from build123d import *

# Parameters (mm, degrees)
BOSS_EXTRU_1_DEPTH = 50
CONG_1_R           = 0.75
CONG_2_R           = 0.25
CONG_3_R           = 0.25


with BuildPart() as part:
    # Esquisse1 → Boss.-Extru.1 (new body)
    with BuildSketch(Plane.XY):
        Polygon((3.2, 0), (0, 0), (0, 8), (-2, 8), (-2, 0), (-2, -2), (5.2, -2), (5.2, 0), (5.2, 8), (3.2, 8), align=None)
    extrude(amount=BOSS_EXTRU_1_DEPTH)

    # Congé1
    cong_1_edges = [part.edges().sort_by_distance(p)[0] for p in [
        (5.2, 8, 25),
        (-2, 8, 25),
    ]]
    fillet(cong_1_edges, radius=CONG_1_R)

    # Congé2
    cong_2_edges = [part.edges().sort_by_distance(p)[0] for p in [
        (3.2, 8, 25),
        (0, 8, 25),
    ]]
    fillet(cong_2_edges, radius=CONG_2_R)

    # Congé3
    cong_3_edges = [part.edges().sort_by_distance(p)[0] for p in [
        (1.6, 0, 0),
        (5.2, 2.625, 0),
        (0, 3.875, 0),
        (5.2, 2.625, 50),
        (-2, 2.625, 0),
        (-2, 2.625, 50),
        (3.95, 8, 0),
        (4.980330086, 7.780330086, 0),
        (-1.780330086, 7.780330086, 0),
        (3.95, 8, 50),
        (4.980330086, 7.780330086, 50),
        (-1.780330086, 7.780330086, 50),
        (1.6, 0, 50),
        (-0.75, 8, 0),
        (-0.75, 8, 50),
        (3.2, 3.875, 0),
        (3.273223305, 7.926776695, 0),
        (-0.073223305, 7.926776695, 0),
        (3.2, 3.875, 50),
        (3.273223305, 7.926776695, 50),
        (-0.073223305, 7.926776695, 50),
        (0, 3.875, 50),
    ]]
    fillet(cong_3_edges, radius=CONG_3_R)


solid = part.part
Geometry check sheet. Reference: the model listing, model coordinates, mm. A direction names the side the tool comes from. Give positions to 0.01 mm unless a question says otherwise; leave off trailing zeros. Order: outer loops, then holes, each group sorted by start corner. A loop starts at its lowest first (then second) coordinate and runs counter-clockwise, first axis right, second up.
1. Draft check along X on faces 3 (the face through (5.2, 3, 25)), 4 (the face through (3.2, 4, 25)), 5 (the face through (-2, 3, 25)), 6 (the face through (2, -2, 25)). Enter one of: pulls with the +X half, pulls with the -X half, needs draft (parallel to the pull), parting line crosses it, or undercut.
Completed:
face 3: pulls with the +X half
face 4: undercut
face 5: pulls with the -X half
face 6: needs draft
2. Sectioned sample at B-B (z = 3). Record the boundary of the cut face in (x, y).
Completed:
outline: (-2, -2) - (5.2, -2) - (5.2, 7.25) arc R0.75 ccw to (4.45, 8) - (3.45, 8) arc R0.25 ccw to (3.2, 7.75) - (3.2, 0) - (0, 0) - (0, 7.75) arc R0.25 ccw to (-0.25, 8) - (-1.25, 8) arc R0.75 ccw to (-2, 7.25) - close
3. Sectioned sample at C-C (x = 2.5). Record the boundary of the cut face in (y, z), then the cut area to 4 significant figures.
Completed:
outline: (-2, 0) - (-0.25, 0) arc R0.25 ccw to (0, 0.25) - (0, 49.75) arc R0.25 ccw to (-0.25, 50) - (-2, 50) - close
area: 100.0 mm2
4. Scan lines: line 1 (X direction, y = 0.25, z = 34.5); line 2 (Y direction, x = 2, z = 17.5); line 3 (Y direction, x = 4.5, z = 29.5). Record each from-to range of solid material in increasing order.
Completed:
line 1: x = -2 to 0, 3.2 to 5.2
line 2: y = -2 to 0
line 3: y = -2 to 8
5. Access from +Z, -Z, +X, -X, +Y, -Y to the whole of each face (thin tool, end or side, straight path). Record for faces 1 (the face through (-1, 8, 25)), 2 (the face through (0, 4, 25)).
Completed:
face 1: +Z, -Z, +X, -X, +Y
face 2: +Z, -Z, +Y
6. Sectioned sample at A-A (y = 4.5). Record the boundary of the cut face in (x, z), then the cut area to 3 significant figures.
Completed:
outline: (-2, 0.25) arc R0.25 ccw to (-1.75, 0) - (-0.25, 0) arc R0.25 ccw to (0, 0.25) - (0, 49.75) arc R0.25 ccw to (-0.25, 50) - (-1.75, 50) arc R0.25 ccw to (-2, 49.75) - close; (3.2, 0.25) arc R0.25 ccw to (3.45, 0) - (4.95, 0) arc R0.25 ccw to (5.2, 0.25) - (5.2, 49.75) arc R0.25 ccw to (4.95, 50) - (3.45, 50) arc R0.25 ccw to (3.2, 49.75) - close
area: 200 mm2
